from build123d import *

# Parameters (mm, degrees)
BASE_EXTRUDE_DEPTH = 3


with BuildPart() as part:
    # Sketch1 → Base-Extrude (new body)
    with BuildSketch(Plane.XY):
        with BuildLine():
            Line((1209.451820501, 108.09887988), (1211.233559267, 105.974449758))
            Line((1211.233559267, 105.974449758), (1210.568605008, 103.078332754))
            Line((1210.568605008, 103.078332754), (1198.969787726, 94.887573091))
            ThreePointArc((1198.969787726, 94.887573091), (1199.754979333, 90.590746745), (1197.058986008, 87.154053204))
            ThreePointArc((1197.058986008, 87.154053204), (1199.345903518, 84.086132658), (1202.705960658, 82.255246482))
            ThreePointArc((1202.705960658, 82.255246482), (1209.850323306, 74.816142589), (1208.153154203, 64.64255908))
            ThreePointArc((1208.153154203, 64.64255908), (1209.513439683, 63.663584022), (1210.741786407, 62.523437946))
            ThreePointArc((1210.741786407, 62.523437946), (1211.288328706, 61.27741643), (1210.911264244, 59.970090727))
            Line((1210.911264244, 59.970090727), (1205.547364782, 52.580569169))
            Line((1205.547364782, 52.580569169), (1202.809005818, 53.947443229))
            Line((1202.809005818, 53.947443229), (1205.868102338, 58.222609567))
            Line((1205.868102338, 58.222609567), (1203.428362014, 59.968366467))
            Line((1203.428362014, 59.968366467), (1200.451593647, 55.808255846))
            ThreePointArc((1200.451593647, 55.808255846), (1199.171644978, 57.50635778), (1198.80528387, 59.601017254))
            Line((1198.80528387, 59.601017254), (1204.319471793, 67.576551504))
            ThreePointArc((1204.319471793, 67.576551504), (1205.223941879, 73.442636449), (1201.095098665, 77.706633686))
            ThreePointArc((1201.095098665, 77.706633686), (1195.300986917, 81.489736173), (1191.700510295, 87.399064684))
            ThreePointArc((1191.700510295, 87.399064684), (1189.361079278, 92.852732142), (1193.525678388, 97.080206622))
            Line((1193.525678388, 97.080206622), (1206.484161244, 107.948359455))
            Line((1206.484161244, 107.948359455), (1209.451820501, 108.09887988))
        make_face()
    extrude(amount=BASE_EXTRUDE_DEPTH)


solid = part.part
Read the model definition and answer for the solid it produces. Units are mm, in the model's axes. A direction names the side the tool comes from. Give positions to 0.01 mm unless a question says otherwise; leave off trailing zeros. Write each loop counter-clockwise with the first axis right and the second up, starting at its lowest first coordinate (ties: lowest second). Pieces come first, ordered by that corner, then holes. Notation, with made-up numbers: (-23.5, 18) - (-1.5, 18) arc R23 ccw to (-1.5, 40) - close; hole circle Ø9 at (9, 17). An arc over 180 degrees is marked (long way). Return JSON: item names as keys, results as strings.
Q1. For faces 1 (the face through (1209.495, 63.678, 1.479)), 2 (the face through (1207.947, 108.023, 1.479)), 3 (the face through (1201.5, 63.5, 1.5)), 4 (the face through (1201.961, 57.917, 1.479)), determine the directions among +Z, -Z, +X, -X, +Y, -Y from which every point of the face is accessible in a straight line to the end or side of a thin tool.
Reply:
{"face 1": "+Z, -Z, +X", "face 2": "+Z, -Z, -X, +Y", "face 3": "+Z, -Z, -X", "face 4": "+Z, -Z"}
Q2. A cutting plane is placed at D-D, the plane x = 1196.25. Determine the outline of the cut face in (y, z), and give its area (3 significant figures).
Reply:
{"outline": "(80.59, 0) - (99.37, 0) - (99.37, 3) - (80.59, 3) - close", "area": "56.3 mm²"}
Q3. For a pull along X with two mould halves and no side action, classify faces 5 (the face through (1205.25, 73.36, 1.48)), 6 (the face through (1204.67, 59.08, 1.48)), 7 (the face through (1199.31, 84.12, 1.48)) as released by +X, released by -X, zero draft, split by the parting line, or undercut.
Reply:
{"face 5": "released by -X", "face 6": "undercut", "face 7": "released by +X"}
Q4. A cutting plane is placed at A-A, the plane z = 1.8. Determine the outline of the cut face in (x, y).
Reply:
{"outline": "(1191.7, 87.4) arc R15.67 ccw to (1201.1, 77.71) arc R6.67 cw to (1204.32, 67.58) - (1198.81, 59.6) arc R4.54 ccw to (1200.45, 55.81) - (1203.43, 59.97) - (1205.87, 58.22) - (1202.81, 53.95) - (1205.55, 52.58) - (1210.91, 59.97) arc R2 ccw to (1210.74, 62.52) arc R13.49 ccw to (1208.15, 64.64) arc R11.49 ccw to (1202.71, 82.26) arc R8.94 cw to (1197.06, 87.15) arc R5.32 ccw to (1198.97, 94.89) - (1210.57, 103.08) - (1211.23, 105.97) - (1209.45, 108.1) - (1206.48, 107.95) - (1193.53, 97.08) arc R5.32 ccw to start"}
Q5. Given P1, Ø5, axis at x = 1208.5, y = 63, coming from the -Z side; P2, Ø1, axis at y = 75, z = 2.5, coming from the -X side; P3, Ø1.5, axis at x = 1197, z = 1, coming from the +Y side, each flat-ended and moving along its own axis, determine where each tip first touches the part or whether it passes through.
Reply:
{"P1": "z = 0", "P2": "x = 1204.14", "P3": "y = 100.62"}
Q6. Consider line 1 along Y through (x, z) = (1201.5, 2.7); line 2 along Y through (x, z) = (1203.5, 0.4); line 3 along Y through (x, z) = (1204.25, 0.45). Determine where each line is inside the solid, lowest interval first. Write a range as [from, to].
Reply:
{"line 1": "[57.27, 63.5], [77.55, 82.7], [96.67, 103.77]", "line 2": "[53.6, 54.91], [59.92, 66.39], [76.22, 81.94], [98.09, 105.45]", "line 3": "[53.23, 55.96], [59.38, 67.48], [75.36, 81.58], [98.62, 106.07]"}
Q7. A cutting plane is placed at B-B, the plane x = 1205. Determine the outline of the cut face in (y, z), and give its area (3 significant figures).
Reply:
{"outline": "(52.85, 0) - (57.01, 0) - (57.01, 3) - (52.85, 3) - close; (58.84, 0) - (68.8, 0) - (68.8, 3) - (58.84, 3) - close; (74.04, 0) - (81.14, 0) - (81.14, 3) - (74.04, 3) - close; (99.15, 0) - (106.7, 0) - (106.7, 3) - (99.15, 3) - close", "area": "86.3 mm²"}
Q8. A cutting plane is placed at C-C, the plane y = 99. Determine the outline of the cut face in (x, z).
Reply:
{"outline": "(1195.81, 0) - (1204.79, 0) - (1204.79, 3) - (1195.81, 3) - close"}
